Read the model definition and answer for the solid it produces. Units are mm, in the model's axes. Face numbers are marked on the shaded views. A direction names the side the tool comes from. Give positions to 0.01 mm unless a question says otherwise; leave off trailing zeros. Loops run counter-clockwise (first coordinate to the right, second up) from the corner with the lowest first, then second, coordinate; pieces in that order, holes last. Notation, with made-up numbers: (64, 25.25) - (84, 25.25) arc R25 ccw to (84, 43.25) - close; hole circle Ø7 at (80, 51.25). An arc over 180 degrees is marked (long way). Write each question's results on one line, items separated by ' | '. Start each with the question number.
Q1. Find the intervals of material crossed by line 1 (X direction, y = 1.15, z = -0.5); line 2 (Z direction, x = -12.25, y = 1.1) (3 decimals); line 3 (X direction, y = 0.7, z = -3.5) (3 decimals), in increasing order. Write a range as from..to.
Q2. The part is cut by section B-B, the plane z = -5. Write down the section's boundary in (x, y) (3 decimals), plus the area to 3 significant figures.
Q3. The part is cut by section D-D, the plane z = 2.5. Write down the section's boundary in (x, y).
Q4. For the marked faces 5, 6 and 7, determine the directions among +Z, -Z, +X, -X, +Y, -Y from which every point of the face is accessible in a straight line to the end or side of a thin tool.
Q5. Given pin 1 (1.5 mm diameter, centred on x = -12.5, z = 0, fed in from -Y) (3 decimals); pin 2 (0.9 mm diameter, centred on y = 0, z = -4, fed in from -X) (3 decimals); pin 3 (0.9 mm diameter, centred on y = -0.5, z = -5, fed in from +X) (3 decimals); pin 4 (0.5 mm diameter, centred on y = 0.5, z = 2, fed in from +X), each flat-ended and moving along its own axis, determine where each tip first touches the part or whether it passes through.
Q6. The part is cut by section C-C, the plane y = -1.05. Write down the section's boundary in (x, z) (3 decimals), plus the area to 3 significant figures.
Q7. Determine the mould class of the marked faces 1, 2, 3 and 4 for opening direction X: +X half, -X half, draft (parallel to the pull), parting line (faces both ways), or undercut.
Q8. The part is cut by section A-A, the plane x = 0.5. Write down the section's boundary in (y, z) (3 decimals).
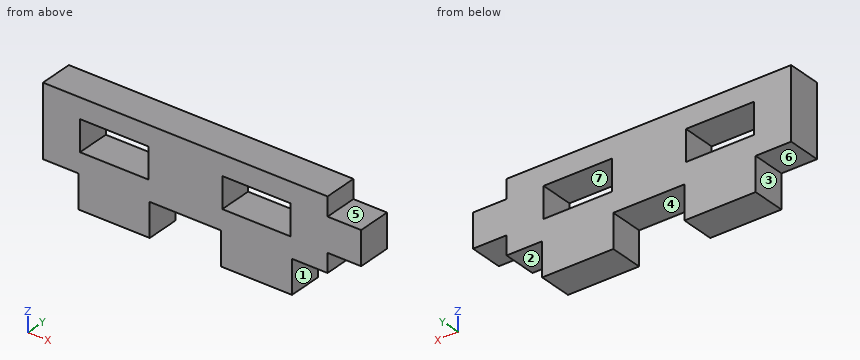
```python
from build123d import *

# Parameters (mm, degrees)
SKETCH1_W           = 6.096
SKETCH1_H           = 2.745994
BOSS_EXTRUDE1_DEPTH = 1.5


with BuildPart() as part:
    # Sketch1 → Boss-Extrude1 (new, symmetric)
    with BuildSketch(Plane(origin=(0, 0, 0), x_dir=(1, 0, 0), z_dir=(0, 1, 0))):
        Polygon((3.175, 3.175), (6.35, 3.175), (6.35, 1.5), (9.35, 1.5), (9.35, -1.5), (6.35, -1.5), (6.35, -3.175), (-6.35, -3.175), (-19.05, -3.175), (-19.05, 3.175), (-15.875, 3.175), (-15.875, 6.175), (-9.525, 6.175), (-9.525, 3.175), (-6.35, 3.175), (-3.175, 3.175), (-3.175, 6.175), (3.175, 6.175), align=None)
        Rectangle(SKETCH1_W, SKETCH1_H, mode=Mode.SUBTRACT)
        with Locations((-12.7, 0)):
            Rectangle(SKETCH1_W, SKETCH1_H, mode=Mode.SUBTRACT)
    extrude(amount=BOSS_EXTRUDE1_DEPTH, both=True)


solid = part.part
```
Check sheet entries:
1) line 1: x = -19.05..-15.75, -9.65..-3.05, 3.05..9.35 | line 2: z = -6.175..-1.373, 1.373..3.175 | line 3: x = -15.875..-9.525, -3.175..3.175
2) outline: (-15.875, -1.5) - (-9.525, -1.5) - (-9.525, 1.5) - (-15.875, 1.5) - close; (-3.175, -1.5) - (3.175, -1.5) - (3.175, 1.5) - (-3.175, 1.5) - close | area: 38.1 mm^2
3) outline: (-19.05, -1.5) - (6.35, -1.5) - (6.35, 1.5) - (-19.05, 1.5) - close
4) face 5: +Z, +X, +Y, -Y | face 6: -Z, -X, +Y, -Y | face 7: +Y, -Y
5) pin 1: passes through | pin 2: stops at x = -15.875 | pin 3: stops at x = 3.175 | pin 4: stops at x = 6.35
6) outline: (-19.05, -3.175) - (-15.875, -3.175) - (-15.875, -6.175) - (-9.525, -6.175) - (-9.525, -3.175) - (-3.175, -3.175) - (-3.175, -6.175) - (3.175, -6.175) - (3.175, -3.175) - (6.35, -3.175) - (6.35, -1.5) - (9.35, -1.5) - (9.35, 1.5) - (6.35, 1.5) - (6.35, 3.175) - (-19.05, 3.175) - close; hole (-15.748, -1.373) - (-9.652, -1.373) - (-9.652, 1.373) - (-15.748, 1.373) - close; hole (-3.048, -1.373) - (3.048, -1.373) - (3.048, 1.373) - (-3.048, 1.373) - close | area: 175 mm^2
7) face 1: +X half | face 2: draft | face 3: -X half | face 4: undercut
8) outline: (-1.5, -6.175) - (1.5, -6.175) - (1.5, -1.373) - (-1.5, -1.373) - close; (-1.5, 1.373) - (1.5, 1.373) - (1.5, 3.175) - (-1.5, 3.175) - close
